from build123d import *

# Parameters (mm, degrees)
SKETCH_1_W             = 405
SKETCH_1_H             = 205
SM_BASE_FLANGE_1_DEPTH = 10
CHAMFER_1_SIZE         = 8
CHAMFER_1_SIZE2        = 5.601660306
CHAMFER_2_SIZE         = 8
CHAMFER_2_SIZE2        = 5.601660306


# Sheet-metal steps are written as plain solids
with BuildPart() as part:
    # Sketch 1 → 基体-法兰1 (new body)
    with BuildSketch(Plane.XY):
        Rectangle(SKETCH_1_W, SKETCH_1_H)
    extrude(amount=-SM_BASE_FLANGE_1_DEPTH)

    # 倒角1
    chamfer_1_edges = [part.edges().sort_by_distance(p)[0] for p in [
        (0, 102.5, -10),
    ]]
    chamfer_1_side = [part.faces().sort_by_distance(p)[0] for p in [
        (0, 102.5, -5),
    ]]
    chamfer(chamfer_1_edges, length=CHAMFER_1_SIZE, length2=CHAMFER_1_SIZE2, reference=chamfer_1_side[0])

    # 倒角2
    chamfer_2_edges = [part.edges().sort_by_distance(p)[0] for p in [
        (0, -102.5, -10),
    ]]
    chamfer_2_side = [part.faces().sort_by_distance(p)[0] for p in [
        (0, -102.5, -5),
    ]]
    chamfer(chamfer_2_edges, length=CHAMFER_2_SIZE, length2=CHAMFER_2_SIZE2, reference=chamfer_2_side[0])


solid = part.part
Verification items for the finished model (mm, model axes). Give positions to 0.01 mm unless a question says otherwise; leave off trailing zeros. Order: outer loops, then holes, each group sorted by start corner. A loop starts at its lowest first (then second) coordinate and runs counter-clockwise, first axis right, second up. Notation, with made-up numbers: M 6,86.5 L 30,86.5 A19 cw 30,110.5 Z; hole C 31.25,0.5 d8. An arc over 180 degrees is marked long. Use one line per item in the form item = value. Start each with the question number.
Q1. Section check A-A (x = -21.5). Enter the section's corners in (y, z), then the cut area to 3 significant figures.
Q2. Scan lines: line 1 along Y through (x, z) = (-74.5, -3.5); line 2 along Y through (x, z) = (-57, -2.5). Record each from-to range of solid material in increasing order. Write a range as [from, to].
Q3. Section check B-B (z = -4.25). Enter the section's corners in (x, y).
Q4. Go/stop test with a flat-tipped pin: pin 1 Ø10 at (x, y) = (32, -73.5) entering from +Z. Record where the tip stops, or that it passes through.
Evaluation:
q1.outline = M -102.5,-2 L -96.9,-10 L 96.9,-10 L 102.5,-2 L 102.5,0 L -102.5,0 Z
q1.area = 2,010 mm2
q2.line_1 = [-101.45, 101.45]
q2.line_2 = [-102.15, 102.15]
q3.outline = M -202.5,-100.92 L 202.5,-100.92 L 202.5,100.92 L -202.5,100.92 Z
q4.pin_1 = 0
